Geometry check sheet. Reference: the model listing, model coordinates, mm. Face numbers are marked on the shaded views. A direction names the side the tool comes from. Give positions to 0.01 mm unless a question says otherwise; leave off trailing zeros. Order: outer loops, then holes, each group sorted by start corner. A loop starts at its lowest first (then second) coordinate and runs counter-clockwise, first axis right, second up. Notation, with made-up numbers: M -36,32 L -17,32 A19 cw -17,61 Z; hole C -10,-18 d9. An arc over 180 degrees is marked long. One line per question, with ' | ' between items. Start each with the question number.
from build123d import *


with BuildPart() as part:
    # Sketch1 → Revolve1 (revolve)
    with BuildSketch(Plane(origin=(0, 0, 0), x_dir=(0, 0, -1), z_dir=(1, 0, 0)), mode=Mode.PRIVATE) as revolve1_sk:
        with BuildLine():
            Line((0.51, 0), (0.51, -18.54))
            Line((0.51, -18.54), (0, -18.54))
            Line((0, -18.54), (0, -24.72))
            Line((0, -24.72), (0.455, -24.72))
            Line((0.455, -24.72), (0.455, -29.72))
            Line((0.455, -29.72), (0.595, -29.72))
            Line((0.595, -29.72), (0.595, -24.72))
            Line((0.595, -24.72), (0.66, -24.56))
            Line((0.66, -24.56), (0.66, -7.62))
            ThreePointArc((0.66, -7.62), (0.735, -7.12), (0.66, -6.62))
            Line((0.66, -6.62), (0.66, 0))
            Line((0.66, 0), (0.51, 0))
        make_face()
    revolve(revolve1_sk.sketch.rotate(Axis((0, -18.54, 0), (0, -1, 0)), 180), axis=Axis((0, -18.54, 0), (0, -1, 0)))


solid = part.part
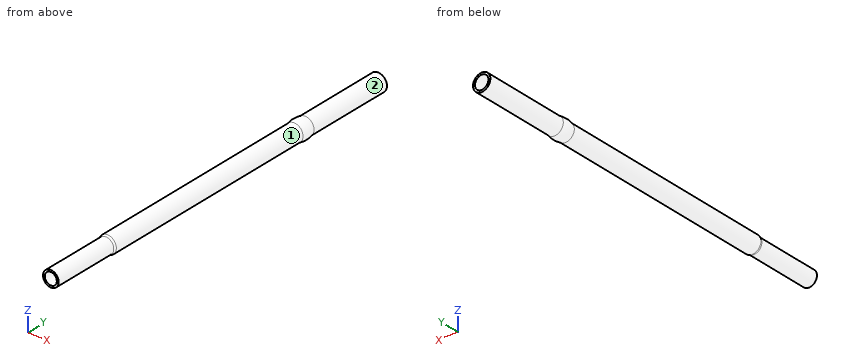
Item 1: Cross-section at B-B, the plane y = -23. Record the cut outline in (x, z), plus the area to 3 significant figures.
Item 2: Material ranges on line 1 along Z through (x, y) = (0.05, -8); line 2 along Z through (x, y) = (-0.4, -2.5); line 3 along X through (y, z) = (-2, 0.1), recorded low to high.
Item 3: Set-up check for the marked faces 1 and 2: record each of +Z, -Z, +X, -X, +Y, -Y from which the full face is reachable in a straight line by a thin tool's end or side.
Item 4: Cross-section at A-A, the plane y = -13.75. Record the cut outline in (x, z), plus the area to 3 significant figures.
Outcome:
1) outline: C 0,0 d1.32 | area: 1.37 mm²
2) line 1: z = -0.66 to -0.51, 0.51 to 0.66 | line 2: z = -0.52 to -0.32, 0.32 to 0.52 | line 3: x = -0.65 to -0.5, 0.5 to 0.65
3) face 1: -Y | face 2: +Y
4) outline: C 0,0 d1.32; hole C 0,0 d1.02 | area: 0.551 mm²
